Could you check a few things on this model? Use its own coordinates, in mm. Coordinates: 2 decimals unless noted, no trailing zeros. Loops run counter-clockwise (first coordinate to the right, second up) from the corner with the lowest first, then second, coordinate; pieces in that order, holes last. Notation, with made-up numbers: (-9.75, 8) -> (1.25, 8) arc R33 cw to (1.25, 47) -> close; hole circle Ø7 at (18.5, -9.75). An arc over 180 degrees is marked (long way). One line per question, with ' | ' between items. Start each with the question number.
(1) I'm going to push flat-ended pins straight in: pin 1 Ø4 at (x, z) = (36, 14.5) entering from +Y; pin 2 Ø1 at (x, z) = (-24.5, 13) entering from -Y; pin 3 Ø1.5 at (x, z) = (-34.5, 24) entering from +Y. Where does each tip first touch, or does it pass through?
(2) Suppose I cut it at B-B (x = 0). Please give me the cut outline in (y, z), plus the area to 3 significant figures.
(3) Suppose I cut it at D-D (z = 13.5). Please give me the cut outline in (x, y).
(4) If I drill on line 1 along Y through (x, z) = (0, 31); line 2 along Y through (x, z) = (33, 37.5); line 3 along X through (y, z) = (9.5, 34), over which ranges is the centre line in solid material (lowest first)?
(5) Suppose I cut it at C-C (y = -25.5). Please give me the cut outline in (x, z), plus the area to 3 significant figures.
(6) Suppose I cut it at A-A (y = 0). Please give me the cut outline in (x, z).
Autodesk Inventor part; units mm, degrees
ref_plane "YZ Plane" through (0, 0, 0) normal (1, 0, 0) x (0, 1, 0)
ref_plane "XZ Plane" through (0, 0, 0) normal (0, 1, 0) x (-1, 0, 0)
ref_plane "XY Plane" through (0, 0, 0) normal (0, 0, 1) x (1, 0, 0)
sketch "Sketch1" plane through (0, 0, 0) normal (0, 0, 1) x (1, 0, 0)
  circle A0 centre (0, 0) radius 46.8237
  circle A1 centre (-39.5, 0) radius 1.5
  arc A2 (-39.5, -3) -> (-39.5, 3) centre (-39.5, 0) ccw
  line L0 (-39.5, -3) -> (-45.7254, -3)
  line L1 (-39.5, 3) -> (-45.7254, 3)
  circle A3 centre (39.5, 0) radius 1.5
  arc A4 (39.5, 3) -> (39.5, -3) centre (39.5, 0) ccw
  line L2 (39.5, 3) -> (45.7254, 3)
  line L3 (39.5, -3) -> (45.7254, -3)
  arc A5 (-45.7254, -3) -> (45.7254, -3) centre (0, 0) ccw
  arc A6 (45.7254, 3) -> (-45.7254, 3) centre (0, 0) ccw
  point P0 (0, 0)
extrude "Extrusion1" add sketch "Sketch1" along normal blind 1
sketch "Sketch2" plane through (0, 0, 1) normal (0, 0, 1) x (1, 0, 0)
  circle A0 centre (0, 0) radius 46.8237
  circle A1 centre (0, 0) radius 45.8237
  point P0 (0, 0)
  dimension "d5" = 1
extrude "Extrusion2" add sketch "Sketch2" along normal blind 38
properties part number "frame5"
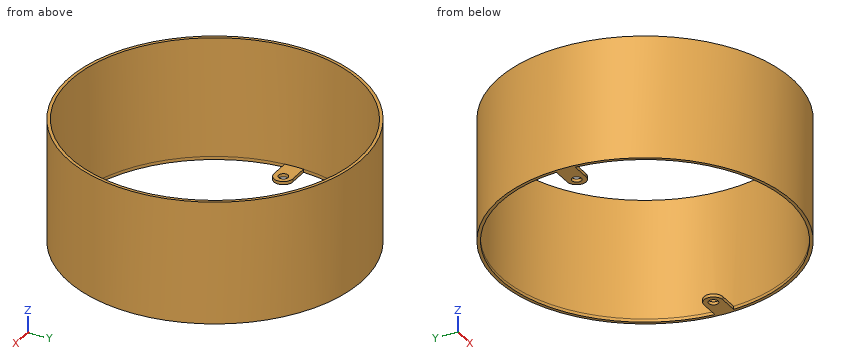
Checks:
1) pin 1: stops at y = 32.19 | pin 2: stops at y = -40.21 | pin 3: stops at y = 32.46
2) outline: (-46.82, 0) -> (-45.82, 0) -> (-45.82, 39) -> (-46.82, 39) -> close; (45.82, 0) -> (46.82, 0) -> (46.82, 39) -> (45.82, 39) -> close | area: 78.0 mm^2
3) outline: circle Ø93.65 at (0, 0); hole circle Ø91.65 at (0, 0)
4) line 1: y = -46.82 to -45.82, 45.82 to 46.82 | line 2: y = -33.22 to -31.79, 31.79 to 33.22 | line 3: x = -45.85 to -44.83, 44.83 to 45.85
5) outline: (-39.27, 0) -> (-38.07, 0) -> (-38.07, 39) -> (-39.27, 39) -> close; (38.07, 0) -> (39.27, 0) -> (39.27, 39) -> (38.07, 39) -> close | area: 93.4 mm^2
6) outline: (-46.82, 0) -> (-41, 0) -> (-41, 1) -> (-45.82, 1) -> (-45.82, 39) -> (-46.82, 39) -> close; (-38, 0) -> (-36.5, 0) -> (-36.5, 1) -> (-38, 1) -> close; (36.5, 0) -> (38, 0) -> (38, 1) -> (36.5, 1) -> close; (41, 0) -> (46.82, 0) -> (46.82, 39) -> (45.82, 39) -> (45.82, 1) -> (41, 1) -> close
